```python
from build123d import *

# Parameters (mm, degrees)
ESQUISSE1_W         = 5
ESQUISSE1_H         = 20.2
BOSS_EXTRU_1_DEPTH  = 22
BOSS_EXTRU_2_DEPTH  = 2
ESQUISSE3_R         = 3.175
BOSS_EXTRU_3_DEPTH  = 7
SKETCH1_W           = 5.2
SKETCH1_H           = 20.2
BOSS_EXTRUDE1_DEPTH = 10
SKETCH2_R           = 1.45
CUT_EXTRUDE1_DEPTH  = 40.785047442
FILLET1_R           = 2


with BuildPart() as part:
    # Esquisse1 → Boss.-Extru.1 (new body)
    with BuildSketch(Plane.XY):
        Rectangle(ESQUISSE1_W, ESQUISSE1_H)
    extrude(amount=BOSS_EXTRU_1_DEPTH)

    # Esquisse2 → Boss.-Extru.2 (add)
    with BuildSketch(Plane.XY.offset(22)):
        with BuildLine():
            Line((2.5, 10.1), (-12.7, 10.1))
            ThreePointArc((-12.7, 10.1), (-22.8, 0), (-12.7, -10.1))
            Line((-12.7, -10.1), (2.5, -10.1))
            Line((2.5, -10.1), (2.5, 10.1))
        make_face()
    extrude(amount=BOSS_EXTRU_2_DEPTH)

    # Esquisse3 → Boss.-Extru.3 (add)
    with BuildSketch(Plane.XY.offset(24)):
        with Locations((-12.7, 0)):
            Circle(ESQUISSE3_R)
    extrude(amount=BOSS_EXTRU_3_DEPTH)

    # Sketch1 → Boss-Extrude1 (add)
    with BuildSketch(Plane(origin=(2.5, 0, 0), x_dir=(0, 0, -1), z_dir=(1, 0, 0))):
        with Locations((-2.6, 0)):
            Rectangle(SKETCH1_W, SKETCH1_H)
    extrude(amount=BOSS_EXTRUDE1_DEPTH)

    # Sketch2 → Cut-Extrude1 (cut, through all)
    with BuildSketch(Plane(origin=(0, 0, 0), x_dir=(-1, 0, 0), z_dir=(0, 0, -1))):
        with Locations((-8.5, -5)):
            Circle(SKETCH2_R)
        with Locations((-8.5, 5)):
            Circle(SKETCH2_R)
    extrude(amount=-CUT_EXTRUDE1_DEPTH, mode=Mode.SUBTRACT)

    # Fillet1
    fillet1_edges = [part.edges().sort_by_distance(p)[0] for p in [
        (2.5, 0, 5.2),
    ]]
    fillet(fillet1_edges, radius=FILLET1_R)


solid = part.part
```
Check sheet for the modelled part. Datum: model origin and axes. Units: mm. A direction names the side the tool comes from. Coordinates: 2 decimals unless noted, no trailing zeros. Order: outer loops, then holes, each group sorted by start corner. A loop starts at its lowest first (then second) coordinate and runs counter-clockwise, first axis right, second up. Notation, with made-up numbers: (82.25, -30.75) -> (87.25, -30.75) arc R6 cw to (87.25, -26.75) -> close; hole circle Ø7 at (-14.5, -14.75). An arc over 180 degrees is marked (long way). Write item = value, one per line. Start each with the question number.
1) Mould release check, pull along Y, two halves, no side actions. Record for faces 6 (the cylindrical face through (9.95, -4.94, 2.56)), 7 (the cylindrical face through (3.1, 0.14, 5.77)), 8 (the flat face through (2, -10.1, 10)): +Y half, -Y half, draft (parallel to the pull), parting line (faces both ways), or undercut.
2) Cross-section at D-D (y = 0). Enter the section's corners in (x, z) (3 decimals).
3) Cross-section at B-B (z = 3). Enter the section's corners in (x, y), then the cut area to 3 significant figures.
4) Go/stop test with flat-tipped pins: P1, Ø3.5, axis at x = 8.5, y = 5, coming from the +Z side; P2, Ø2, axis at x = -14.5, y = 4, coming from the -Z side; P3, Ø6, axis at y = 6.5, z = 23.5, coming from the -X side. Record where each tip stops, or that it passes through.
5) Material ranges on L1, parallel to Y at x = 8.5, z = 2.7; L2, parallel to X at y = 5.75, z = 19.5; L3, parallel to Z at x = -7.5, y = 3.25, recorded low to high.
6) Cross-section at C-C (y = 5.5). Enter the section's corners in (x, z).
7) Access from +Z, -Z, +X, -X, +Y, -Y to the whole of each face (thin tool, end or side, straight path). Record for faces 1 (the flat face through (2, 10.1, 10)), 2 (the cylindrical face through (-9.67, 0.95, 27.45)), 3 (the cylindrical face through (-22.8, 0.2, 23)), 4 (the flat face through (8, 0, 5.2)), 5 (the flat face through (-2.5, 0, 11)).
8) Cross-section at A-A (x = 8.5). Enter the section's corners in (y, z).
Ans:
q1.face_6 = undercut
q1.face_7 = draft
q1.face_8 = -Y half
q2.outline = (-22.8, 22) -> (-2.5, 22) -> (-2.5, 0) -> (12.5, 0) -> (12.5, 5.2) -> (4.5, 5.2) arc R2 cw to (2.5, 7.2) -> (2.5, 24) -> (-9.525, 24) -> (-9.525, 31) -> (-15.875, 31) -> (-15.875, 24) -> (-22.8, 24) -> close
q3.outline = (-2.5, -10.1) -> (12.5, -10.1) -> (12.5, 10.1) -> (-2.5, 10.1) -> close; hole circle Ø2.9 at (8.5, -5); hole circle Ø2.9 at (8.5, 5)
q3.area = 290 mm²
q4.P1 = 5.2
q4.P2 = 22
q4.P3 = -22.17
q5.L1 = -10.1 to -6.45, -3.55 to 3.55, 6.45 to 10.1
q5.L2 = -2.5 to 2.5
q5.L3 = 22 to 24
q6.outline = (-21.17, 22) -> (-2.5, 22) -> (-2.5, 0) -> (7.14, 0) -> (7.14, 5.2) -> (4.5, 5.2) arc R2 cw to (2.5, 7.2) -> (2.5, 24) -> (-21.17, 24) -> close; (9.86, 0) -> (12.5, 0) -> (12.5, 5.2) -> (9.86, 5.2) -> close
q7.face_1 = +Z, -Z, +X, -X, +Y
q7.face_2 = +Z
q7.face_3 = +Z, -Z, -X
q7.face_4 = +Z, +X, +Y, -Y
q7.face_5 = -Z, -X, +Y, -Y
q8.outline = (-10.1, 0) -> (-6.45, 0) -> (-6.45, 5.2) -> (-10.1, 5.2) -> close; (-3.55, 0) -> (3.55, 0) -> (3.55, 5.2) -> (-3.55, 5.2) -> close; (6.45, 0) -> (10.1, 0) -> (10.1, 5.2) -> (6.45, 5.2) -> close
